Could you check a few things on this model? Use its own coordinates, in mm. Face numbers are marked on the shaded views. A direction names the side the tool comes from. Coordinates: 2 decimals unless noted, no trailing zeros. Order: outer loops, then holes, each group sorted by start corner. A loop starts at its lowest first (then second) coordinate and runs counter-clockwise, first axis right, second up.
Autodesk Inventor part; units mm, degrees
ref_plane "YZ Plane" through (0, 0, 0) normal (1, 0, 0) x (0, 1, 0)
ref_plane "XZ Plane" through (0, 0, 0) normal (0, 1, 0) x (-1, 0, 0)
ref_plane "XY Plane" through (0, 0, 0) normal (0, 0, 1) x (1, 0, 0)
sketch "Эскиз1" plane through (0, 0, 0) normal (1, 0, 0) x (0, 1, 0)
  line L0 (0, 0) -> (4, 0)
  line L1 (4, 0) -> (4, -125)
  line L2 (4, -125) -> (0, -125)
  line L3 (0, -125) -> (0, 0)
  dimension "d0" = 4
  dimension "d1" = 125
extrude "Выдавливание1" add sketch "Эскиз1" along normal blind 20
sketch "Эскиз2" plane through (0, 0, 0) normal (0, 0, 1) x (1, 0, 0)
  line L0 (0, 0) -> (0, 4)
  line L1 (0, 4) -> (-20.6542, 14.0196)
  line L2 (-20.6542, 14.0196) -> (-22.225, 10.7816)
  line L3 (-22.225, 10.7816) -> (0, 0)
  line L4 (0, 4) -> (20, 4)
  line L5 (0, 0) -> (20, 0)
  line L6 (10, 4) -> (10, 0)
  line L7 (20, 4) -> (40.6542, 14.0196)
  line L8 (40.6542, 14.0196) -> (42.225, 10.7816)
  line L9 (42.225, 10.7816) -> (20, 0)
extrude "Выдавливание2" add sketch "Эскиз2" against normal blind 20 contours L3 L2 L1 L0 | L6 L4 L7 L8 L9 L5
sketch "Эскиз3" plane through (20, 0, 0) normal (1, 0, 0) x (0, 0, -1)
  circle A0 centre (114.9699, 1.5875) radius 9.6564
  line L0 (125, 0) -> (125, 4)
  point P0 (0, 0)
  dimension "d16" = 10.0301
extrude "Выдавливание3" add sketch "Эскиз3" against normal blind 20
sketch "Эскиз4" plane through (0, 0, -20) normal (0, 0, -1) x (-1, 0, 0)
  line L0 (-20, 4) -> (-20, 0)
  line L1 (-20, 4) -> (-40.6542, 14.0196)
  line L2 (-40.6542, 14.0196) -> (-42.225, 10.7816)
  line L3 (-42.225, 10.7816) -> (-20, 0)
  line L4 (-40.6542, 14.0196) -> (-37.955, 12.7102)
  line L5 (-37.955, 12.7102) -> (-39.5258, 9.4722)
  line L6 (-42.225, 10.7816) -> (-39.5258, 9.4722)
  line L7 (-42.225, 10.7816) -> (-40.6542, 14.0196)
  line L8 (20.6542, 14.0196) -> (0, 4)
  line L9 (0, 0) -> (0, 4)
  line L10 (0, 0) -> (22.225, 10.7816)
  line L11 (22.225, 10.7816) -> (20.6542, 14.0196)
  line L12 (20.6542, 14.0196) -> (17.955, 12.7102)
  line L13 (17.955, 12.7102) -> (19.5258, 9.4722)
  line L14 (19.5258, 9.4722) -> (22.225, 10.7816)
  line L15 (20.6542, 14.0196) -> (22.225, 10.7816)
  dimension "d8" = 3
  dimension "d9" = 3
extrude "Выдавливание4" add sketch "Эскиз4" along normal up to surface (105 mm away) contours L5 L3 L2 L1 | L11 L10 L13 L8
sketch "Эскиз5" plane through (39.5258, 9.4722, -125) normal (0, 0, -1) x (-0.8997207, -0.436466, 0)
  line L0 (0, 3.5989) -> (0, 0)
  line L1 (0, 0) -> (21.7021, 0)
  line L2 (19.9562, 3.5989) -> (21.7021, 0)
  line L3 (19.9562, 3.5989) -> (0, 3.5989)
  line L4 (53.13, 25.7741) -> (50.3035, 28.0017)
  line L5 (50.3035, 28.0017) -> (37.9507, 12.3282)
  line L6 (39.6965, 8.7293) -> (37.9507, 12.3282)
  line L7 (39.6965, 8.7293) -> (53.13, 25.7741)
  line L8 (53.13, 25.7741) -> (50.3035, 28.0017)
  line L9 (54.987, 28.1302) -> (53.13, 25.7741)
  line L10 (52.1605, 30.3579) -> (54.987, 28.1302)
  line L11 (50.3035, 28.0017) -> (52.1605, 30.3579)
  line L12 (0, 3.5989) -> (0, 0)
  line L13 (-3, 3.5989) -> (0, 3.5989)
  line L14 (-3, 0) -> (-3, 3.5989)
  line L15 (0, 0) -> (-3, 0)
extrude "Выдавливание5" add sketch "Эскиз5" against normal blind 20 contours L3 L2 L1 L0 | L7 L6 L5 L4
sketch "Эскиз6" plane through (0, 4, 0) normal (0, 1, 0) x (1, 0, 0)
  line L0 (0, 105.6197) -> (0, 105)
  line L1 (0, 105) -> (0, 20)
  line L2 (0, 20) -> (0, 0)
  line L3 (0, 0) -> (20, 0)
  line L4 (20, 20) -> (20, 0)
  line L5 (20, 105) -> (20, 20)
  line L6 (20, 105.6197) -> (20, 105)
  line L7 (-19.5258, 105) -> (0, 105)
  line L8 (0, 105) -> (20, 105)
  line L9 (0, 20) -> (20, 20)
  line L10 (0, 125) -> (20, 125)
  line L11 (0, 124.3201) -> (20, 124.3201)
  line L12 (20, 125) -> (20, 124.3201)
  line L13 (0, 125) -> (0, 124.3201)
  line L14 (20, 105.6197) -> (0, 105.6197)
  point P0 (0, 0)
extrude "Выдавливание6" cut sketch "Эскиз6" against normal blind 20 contours L14 L6 L8 L0 | L8 L5 L9 L1 | L10 L12 L11 L13
sketch "Эскиз7" plane through (0, 0, -20) normal (0, -1, 0) x (1, 0, 0)
  line L0 (0, 0) -> (0, 20)
  line L1 (20, 0) -> (20, 20)
  line L2 (0, 20) -> (20, 20)
  line L3 (20, 20) -> (20, 12.7)
  line L4 (20, 12.7) -> (0, 12.7)
  line L5 (0, 12.7) -> (0, 20)
extrude "Выдавливание7" add sketch "Эскиз7" along normal blind 20
sketch "Эскиз8" plane through (0, 0, -105) normal (0, -1, 0) x (1, 0, 0)
  line L0 (20, 97.7) -> (0, 97.7)
  line L1 (0, 97.7) -> (0, 85)
  line L2 (0, 85) -> (0, 0)
  line L3 (0, 0) -> (20, 0)
  line L4 (20, 85) -> (20, 0)
  line L5 (20, 97.7) -> (20, 85)
  line L6 (39.5258, 85) -> (20, 85)
  line L7 (0, 85) -> (-19.5258, 85)
  line L8 (20, 105) -> (42.225, 105)
  line L9 (20, 105) -> (20, 97.7)
  line L10 (20, 97.7) -> (20, 85)
  line L11 (39.5258, 85) -> (20, 85)
  line L12 (39.5258, 85) -> (39.5258, 0)
  line L13 (20, 0) -> (39.5258, 0)
  line L14 (20, -0.6197) -> (20, 0)
  line L15 (20, -19.3201) -> (20, -0.6197)
  line L16 (20, -19.3201) -> (20, -20)
  line L17 (42.225, -20) -> (20, -20)
  line L18 (42.225, 105) -> (42.225, -20)
  line L19 (-22.225, 105) -> (0, 105)
  line L20 (-22.225, 105) -> (-22.225, -20)
  line L21 (-22.225, -20) -> (0, -20)
  line L22 (0, -19.3201) -> (0, -20)
  line L23 (0, -0.6197) -> (0, -19.3201)
  line L24 (0, 0) -> (0, -0.6197)
  line L25 (-19.5258, 0) -> (0, 0)
  line L26 (-19.5258, 85) -> (-19.5258, 0)
  line L27 (0, 85) -> (-19.5258, 85)
  line L28 (0, 97.7) -> (0, 85)
  line L29 (0, 105) -> (0, 97.7)
  line L30 (20, 85) -> (0, 85)
  point P0 (0, 97.7)
extrude "Выдавливание8" cut sketch "Эскиз8" against normal blind 20
sketch "Эскиз9" plane through (20, -20, -7.3) normal (0, 0, -1) x (-1, 0, 0)
  line L0 (-22.225, 25.4) -> (49.2125, 25.4)
  line L1 (49.2125, 25.4) -> (49.2125, 17.4625)
  line L2 (49.2125, 17.4625) -> (-22.225, 17.4625)
  line L3 (-22.225, 17.4625) -> (-22.225, 25.4)
  line L4 (-22.225, 25.4) -> (-9.525, 25.4)
  line L5 (-9.525, 25.4) -> (-9.525, 17.4625)
  line L6 (-9.525, 17.4625) -> (-22.225, 17.4625)
  line L7 (-22.225, 17.4625) -> (-22.225, 25.4)
  line L8 (49.2125, 25.4) -> (39.6875, 25.4)
  line L9 (39.6875, 25.4) -> (39.6875, 17.4625)
  line L10 (39.6875, 17.4625) -> (49.2125, 17.4625)
  line L11 (49.2125, 17.4625) -> (49.2125, 25.4)
  point P0 (20, 20)
extrude "Выдавливание9" add sketch "Эскиз9" along normal blind 110.4875 and the other way blind 10 contours L0 L5 L2 L3 | L0 L1 L2 L9
sketch "Эскиз10" plane through (-19.6875, -2.5375, -117.7875) normal (1, 0, 0) x (0, 0, -1)
  line L0 (-117.7875, -17.4625) -> (-117.7875, 6.5375)
  line L1 (-110.4875, -17.4625) -> (-117.7875, -17.4625)
  line L2 (-110.4875, -17.4625) -> (-110.4875, 6.5375)
  line L3 (-110.4875, 6.5375) -> (-117.7875, 6.5375)
  line L4 (-120.4875, 7.9375) -> (0, 7.9375)
  line L5 (-120.4875, 0) -> (0, 0)
  line L6 (0, 7.9375) -> (-9.525, 7.9375)
  line L7 (-9.525, 7.9375) -> (-9.525, 0)
  line L8 (-9.525, 0) -> (0, 0)
  line L9 (0, 0) -> (0, 7.9375)
  point P0 (-117.7875, 2.5375)
extrude "Выдавливание10" add sketch "Эскиз10" along normal up to surface (49.2125 mm away)
properties part number "ПАЛЬЧИК ножки врозь"
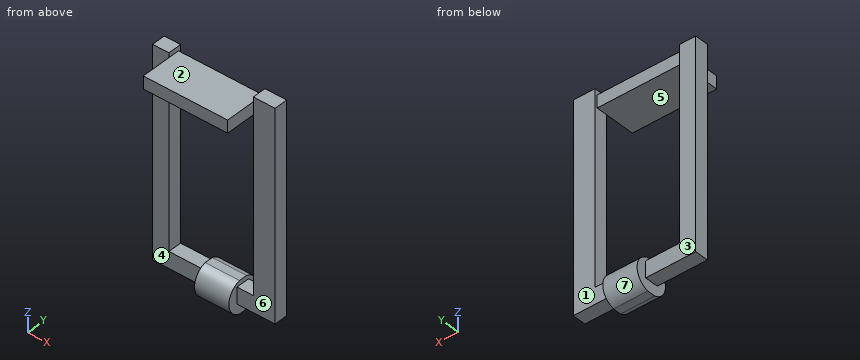
Item 1: Thinking about a two-plate mould opening in Z: for the marked faces 5, 6 and 7, which applies, +Z half, -Z half, draft (parallel to the pull), parting line (faces both ways), or undercut?
Item 2: I need wall thicknesses on line 1 (X direction, y = 0.5, z = -57.5) (1 decimal); line 2 (Y direction, x = 30, z = -20); line 3 (Z direction, x = -1.5, y = 1.5). Which ranges of each line are inside material? Lowest first, please.
Item 3: Which directions (+Z, -Z, +X, -X, +Y, -Y) give clear straight access to the entire face, cutting with the end or side of a thin tool? Please do the marked faces 1, 2, 3 and 4.
Item 4: For pin 1 Ø12 at (x, y) = (1, -13) entering from +Z; pin 2 Ø8 at (y, z) = (-10, -4) entering from -X; pin 3 Ø1 at (x, y) = (12.5, -7) entering from -Z, each with a flat end and sliding along its axis, tell me the tip position at first contact or that it passes through.
Item 5: Suppose I cut it at B-B (z = -99.5). List the corners of the cut face in (x, y) for me (1 decimal), and give its area (3 significant figures).
Item 6: Suppose I cut it at A-A (y = 2.5). List the corners of the cut face in (x, z) for me (1 decimal), and give its area (3 significant figures).
Item 7: Suppose I cut it at D-D (x = 31.5). List the corners of the cut face in (y, z) for me.
Item 8: Suppose I cut it at C-C (x = 10). List the corners of the cut face in (y, z) for me.
Geometry results:
1. face 5: undercut
1. face 6: draft
1. face 7: parting line
2. line 1: x = -29.2 to -19.7, 29.5 to 42.2
2. line 2: y = -2.54 to 5.4
2. line 3: z = -117.79 to -108.26, -7.3 to 0
3. face 1: +Z, -Z, +X, +Y
3. face 2: +Z, +Y, -Y
3. face 3: +Z, -Z, -X, +Y
3. face 4: -Z, -X, -Y
4. pin 1: stops at z = 0
4. pin 2: stops at x = -19.69
4. pin 3: stops at z = -120.25
5. outline: (-29.2, -2.5) - (-19.7, -2.5) - (-19.7, 5.4) - (-29.2, 5.4) - close; (29.5, -2.5) - (42.2, -2.5) - (42.2, 5.4) - (29.5, 5.4) - close
5. area: 176 mm2
6. outline: (-29.2, -117.8) - (0, -117.8) - (0, -124.3) - (20, -124.3) - (20, -117.8) - (42.2, -117.8) - (42.2, 2.7) - (29.5, 2.7) - (29.5, 0) - (-19.7, 0) - (-19.7, 2.7) - (-29.2, 2.7) - close; hole (-19.7, -108.3) - (0, -108.3) - (0, -105.6) - (20, -105.6) - (20, -108.3) - (29.5, -108.3) - (29.5, -7.3) - (-19.7, -7.3) - close
6. area: 3,690 mm2
7. outline: (-2.54, -117.79) - (5.4, -117.79) - (5.4, 2.7) - (-2.54, 2.7) - close
8. outline: (-20, -7.3) - (4, -7.3) - (4, 0) - (-20, 0) - close; (-0.82, -124.32) - (4, -124.32) arc R9.66 ccw to (4, -105.62) - (-0.82, -105.62) arc R9.66 ccw to start
